from build123d import *

# Parameters (mm, degrees)
ESBO_O1_R                = 9
ESBO_O1_R_2              = 4.7625
RESSALTO_EXTRUS_O1_DEPTH = 5
ESBO_O2_R                = 7.75
ESBO_O2_R_2              = 6.25
CORTE_EXTRUS_O1_DEPTH    = 0.5


with BuildPart() as part:
    # Esboço1 → Ressalto-extrusão1 (new body)
    with BuildSketch(Plane.XY):
        Circle(ESBO_O1_R)
        Circle(ESBO_O1_R_2, mode=Mode.SUBTRACT)
    extrude(amount=RESSALTO_EXTRUS_O1_DEPTH)

    # Esboço2 → Corte-extrusão1 (cut)
    with BuildSketch(Plane(origin=(0, 0, 0), x_dir=(-1, 0, 0), z_dir=(0, 0, -1))):
        Circle(ESBO_O2_R)
        Circle(ESBO_O2_R_2, mode=Mode.SUBTRACT)
    corte_extrus_o1 = extrude(amount=-CORTE_EXTRUS_O1_DEPTH, mode=Mode.SUBTRACT)

    # Espelhar2: Corte-extrusão1 across plane
    add(corte_extrus_o1.mirror(Plane.XY.offset(2.5)), mode=Mode.SUBTRACT)


solid = part.part
Could you check a few things on this model? Use its own coordinates, in mm. A direction names the side the tool comes from. Coordinates: 2 decimals unless noted, no trailing zeros. Write each loop counter-clockwise with the first axis right and the second up, starting at its lowest first coordinate (ties: lowest second). Pieces come first, ordered by that corner, then holes. Notation, with made-up numbers: (-35, 76.5) - (21, 76.5) arc R33 ccw to (21, 109.5) - close; hole circle Ø7 at (46.5, 65.25). An arc over 180 degrees is marked (long way). Put each result on its own line as item: value. Start each with the question number.
Q1. Which directions (+Z, -Z, +X, -X, +Y, -Y) give clear straight access to the entire face, cutting with the end or side of a thin tool? Please do faces 1 (the flat face through (-0.5, 6.4, 0.5)), 2 (the cylindrical face through (1.009, 7.684, 4.754)), 3 (the cylindrical face through (-3.78, -2.9, 2.46)).
Q2. Please list where these lines run through material, in increasing order: L1, parallel to Y at x = 0, z = 0.3; L2, parallel to Y at x = 0, z = 1.1; L3, parallel to Y at x = 2.75, z = 1.95.
Q3. Thinking about a two-plate mould opening in Y: for faces 4 (the cylindrical face through (-5.96, 1.88, 0.25)), 5 (the cylindrical face through (-1.172, 8.923, 2.465)), 6 (the flat face through (4, 7, 0)), which applies, pulls with the +Y half, pulls with the -Y half, needs draft (parallel to the pull), parting line crosses it, or undercut?
Q4. I want a section at D-D on y = 7. Write out the boundary of the cut face in (x, z), plus the area to 3 significant figures.
Q5. I want a section at C-C on z = 2.3. Write out the boundary of the cut face in (x, y) (1 decimal), plus the area to 3 significant figures.
Q6. I want a section at B-B on y = 1.5. Write out the boundary of the cut face in (x, z), plus the area to 3 significant figures.
Q7. I want a section at A-A on x = 0. Write out the boundary of the cut face in (y, z).
Q8. I'm going to push flat-ended pins straight in: P1, Ø1.5, axis at x = 7, z = 4, coming from the +Y side; P2, Ø4.5, axis at x = -0.5, y = 2, coming from the +Z side. Where does each tip first touch, or does it pass through?
Checks:
1. face 1: -Z
1. face 2: +Z
1. face 3: +Z, -Z
2. L1: -9 to -7.75, -6.25 to -4.76, 4.76 to 6.25, 7.75 to 9
2. L2: -9 to -4.76, 4.76 to 9
2. L3: -8.57 to -3.89, 3.89 to 8.57
3. face 4: undercut
3. face 5: parting line crosses it
3. face 6: needs draft
4. outline: (-5.66, 0) - (-3.33, 0) - (-3.33, 0.5) - (3.33, 0.5) - (3.33, 0) - (5.66, 0) - (5.66, 5) - (3.33, 5) - (3.33, 4.5) - (-3.33, 4.5) - (-3.33, 5) - (-5.66, 5) - close
4. area: 49.9 mm²
5. outline: circle Ø18 at (0, 0); hole circle Ø9.5 at (0, 0)
5. area: 183 mm²
6. outline: (-8.87, 0) - (-7.6, 0) - (-7.6, 0.5) - (-6.07, 0.5) - (-6.07, 0) - (-4.52, 0) - (-4.52, 5) - (-6.07, 5) - (-6.07, 4.5) - (-7.6, 4.5) - (-7.6, 5) - (-8.87, 5) - close; (4.52, 0) - (6.07, 0) - (6.07, 0.5) - (7.6, 0.5) - (7.6, 0) - (8.87, 0) - (8.87, 5) - (7.6, 5) - (7.6, 4.5) - (6.07, 4.5) - (6.07, 5) - (4.52, 5) - close
6. area: 40.5 mm²
7. outline: (-9, 0) - (-7.75, 0) - (-7.75, 0.5) - (-6.25, 0.5) - (-6.25, 0) - (-4.76, 0) - (-4.76, 5) - (-6.25, 5) - (-6.25, 4.5) - (-7.75, 4.5) - (-7.75, 5) - (-9, 5) - close; (4.76, 0) - (6.25, 0) - (6.25, 0.5) - (7.75, 0.5) - (7.75, 0) - (9, 0) - (9, 5) - (7.75, 5) - (7.75, 4.5) - (6.25, 4.5) - (6.25, 5) - (4.76, 5) - close
8. P1: y = 6.48
8. P2: through
